Solid Edge part; units mm, degrees
sketch "Sketch1" plane through (0, 0, 0) normal (1, 0, 0) x (0, 1, 0)
  line L0 (-15, 0) -> (-15, -10)
  line L1 (-15, -10) -> (8, -10)
  line L2 (8, -10) -> (8, 20)
  line L3 (8, 20) -> (0, 20)
  line L4 (0, 20) -> (0, 0)
  line L5 (0, 0) -> (-15, 0)
  dimension "D1" = 8
  dimension "D2" = 15
extrude "Protrusion1" add sketch "Sketch1" along normal mid plane 22.5
hole "Hole_1" at (0, -7.5, 0) direction (0, 0, -1) diameter 5.5 end up to next start chamfer 0.4 start chamfer angle 45 end chamfer 0.4 end chamfer angle 45
properties material "Polyethylene, low density"
Model file for the job. Use its own axes, mm. A direction names the side the tool comes from. Coordinates: 2 decimals unless noted, no trailing zeros. Write each loop counter-clockwise with the first axis right and the second up, starting at its lowest first coordinate (ties: lowest second). Pieces come first, ordered by that corner, then holes. Notation, with made-up numbers: (-13.75, 36) - (7.25, 36) arc R7 cw to (7.25, 46) - close; hole circle Ø4 at (68, 43.25). An arc over 180 degrees is marked (long way). One line per item, written item: value. Start each with the question number.
1. Slice it at D-D (y = -2). Write the cut outline in (x, z), plus the area to 3 significant figures.
2. Slice it at A-A (y = -7.5). Write the cut outline in (x, z), plus the area to 3 significant figures.
3. Tool access for faces 4 (the flat face through (0, 4, 20)), 5 (the flat face through (-3, -6, 0)): list every direction of +Z, -Z, +X, -X, +Y, -Y with a clear straight run to the whole face (end or side of a thin tool).
4. Probe line 1 (X direction, y = -7.5, z = -4); line 2 (Y direction, x = 0, z = -6.5); line 3 (Z direction, x = -8.5, y = -12.5). List the from-to ranges inside material, lowest first. Write a range as from..to.
5. Mould opens along Y. For faces 1 (the flat face through (0, -4, -10)), 2 (the cylindrical face through (-1.05, -10.04, -4.94)), 3 (the flat face through (0, -15, -5)) say: released by +Y, released by -Y, zero draft, split by the parting line, or undercut.
6. Flat gauge pins, fed straight in: pin 1 (3 mm diameter, centred on x = -1.5, y = -7.5, fed in from +Z); pin 2 (12 mm diameter, centred on x = 2, y = -9, fed in from +Z); pin 3 (10 mm diameter, centred on x = 4, z = 6, fed in from -Y); pin 4 (4.5 mm diameter, centred on x = 0, y = -7.5, fed in from +Z). Where does each tip first touch, or does it go through?
7. Slice it at B-B (x = 0). Write the cut outline in (y, z), plus the area to 3 significant figures.
8. Slice it at C-C (z = 12.25). Write the cut outline in (x, y).
Answers below:
1. outline: (-11.25, -10) - (11.25, -10) - (11.25, 0) - (-11.25, 0) - close
1. area: 225 mm^2
2. outline: (-11.25, -10) - (-3.15, -10) - (-2.75, -9.6) - (-2.75, -0.4) - (-3.15, 0) - (-11.25, 0) - close; (2.75, -9.6) - (3.15, -10) - (11.25, -10) - (11.25, 0) - (3.15, 0) - (2.75, -0.4) - close
2. area: 170 mm^2
3. face 4: +Z, +X, -X, +Y, -Y
3. face 5: +Z, +X, -X, -Y
4. line 1: x = -11.25..-2.75, 2.75..11.25
4. line 2: y = -15..-10.25, -4.75..8
4. line 3: z = -10..0
5. face 1: zero draft
5. face 2: undercut
5. face 3: released by -Y
6. pin 1: stops at z = -0.15
6. pin 2: stops at z = 0
6. pin 3: stops at y = 0
6. pin 4: passes through
7. outline: (-15, -10) - (-10.65, -10) - (-10.25, -9.6) - (-10.25, -0.4) - (-10.65, 0) - (-15, 0) - close; (-4.75, -9.6) - (-4.35, -10) - (8, -10) - (8, 20) - (0, 20) - (0, 0) - (-4.35, 0) - (-4.75, -0.4) - close
7. area: 335 mm^2
8. outline: (-11.25, 0) - (11.25, 0) - (11.25, 8) - (-11.25, 8) - close
